from build123d import *
from build123d.topology import SkipClean

# Parameters (mm, degrees)
BASPROSKE_W      = 3
BASPROSKE_H      = 4.25
TOOTHCUT_DEPTH   = 7.717514421
TEETHCUTS_COUNT  = 15
TEETHCUTS_ANGLE  = 336
HUBNEARONE_START = 2.0000508
HUBNEAONESKE_R   = 3.124
HUBNEARONE_DEPTH = 2.0000508
BORSKE_R         = 1.75
BORE_DEPTH       = 5.0000508


with BuildPart() as part:
    # BasProSke → Base-Revolve (revolve)
    with BuildSketch(Plane(origin=(0, 0, 0), x_dir=(1, 0, 0), z_dir=(0, 1, 0)), mode=Mode.PRIVATE) as base_revolve_sk:
        with Locations((1.5, 2.125)):
            Rectangle(BASPROSKE_W, BASPROSKE_H)
    revolve(base_revolve_sk.sketch.rotate(Axis((-10, 0, 0), (1, 0, 0)), 180), axis=Axis((-10, 0, 0), (1, 0, 0)))

    # TooCutSke → ToothCut (cut, through all)
    with BuildSketch(Plane(origin=(0, 0, 0), x_dir=(0, 0, -1), z_dir=(1, 0, 0))):
        with BuildLine():
            ThreePointArc((0.265767165, 3.112674704), (0, 3.124), (-0.265767165, 3.112674704))
            ThreePointArc((-0.265767165, 3.112674704), (-0.418628877, 3.712626775), (-0.800767345, 4.19974009))
            ThreePointArc((-0.800767345, 4.19974009), (0, 4.2754), (0.800767345, 4.19974009))
            ThreePointArc((0.800767345, 4.19974009), (0.418628877, 3.712626775), (0.265767165, 3.112674704))
        make_face()
    toothcut = extrude(amount=TOOTHCUT_DEPTH, mode=Mode.SUBTRACT)

    # TeethCuts: ToothCut ×15 about axis
    teethcuts_axis = Axis((-10, 0, 0), (1, 0, 0))
    for i in range(1, TEETHCUTS_COUNT):
        add(toothcut.rotate(teethcuts_axis, i * TEETHCUTS_ANGLE / (TEETHCUTS_COUNT - 1)), mode=Mode.SUBTRACT)

    # HubNeaOneSke → HubNearOne (add)
    with SkipClean():  # the faces are left unmerged after this step: merging them gives an invalid solid
        with BuildSketch(Plane.ZY.offset(HUBNEARONE_START)):
            Circle(HUBNEAONESKE_R)
        extrude(amount=-HUBNEARONE_DEPTH)

    # BorSke → Bore (cut, symmetric)
    with SkipClean():  # the faces are left unmerged after this step: merging them gives an invalid solid
        with BuildSketch(Plane(origin=(0, 0, 0), x_dir=(0, 0, -1), z_dir=(1, 0, 0))):
            with Locations(Location((0, 0, 0), (0, 0, 180))):
                Circle(BORSKE_R)
        extrude(amount=BORE_DEPTH, both=True, mode=Mode.SUBTRACT)


solid = part.part
Geometry: final body of the model. Coordinates: model frame, mm. A direction names the side the tool comes from. Give positions to 0.01 mm unless a question says otherwise; leave off trailing zeros. Write each loop counter-clockwise with the first axis right and the second up, starting at its lowest first coordinate (ties: lowest second). Pieces come first, ordered by that corner, then holes.
(1) Cut plane B-B, the plane x = -0.2. Return loops of the section in (y, z).
(2) First-contact query: P1, Ø1.5, axis at x = -1, z = -3, coming from the +Y side; P2, Ø0.5, axis at y = 3, z = 2, coming from the -X side; P3, Ø1, axis at x = 0, y = -3.5, coming from the +Z side. Flat tips, straight axial feed; report the tip coordinate or a pass-through.
(3) Access query for faces 1 (the flat face through (0, 2, 3)), 2 (the cylindrical face through (1.48, -3.54, 1.18)), 3 (the cylindrical face through (1.48, 3.22, -1.89)), 4 (the cylindrical face through (1.48, 2.77, -2.47)), 5 (the cylindrical face through (1.479, -3.711, -0.364)). Directions: +Z, -Z, +X, -X, +Y, -Y. A direction counts if a zero-diameter tool reaches every point of the face in a straight line with its end or side. Return the directions, or none.
(4) Mould query, pull axis Z, two halves, no side actions, for faces 6 (the flat face through (0, -2.4, 2.6)), 7 (the cylindrical face through (1.479, -2.198, 2.992)), 8 (the cylindrical face through (1.48, -3.23, 1.84)). Classes: released by +Z, released by -Z, zero draft, split by the parting line, or undercut.
(5) Ray query, line 1 (Y direction, x = 1.35, z = 3.5); line 2 (Z direction, x = 2.6, y = -3.25); line 3 (Y direction, x = -0.15, z = 0). Return the intervals inside material, ascending.
(6) Cut plane A-A, the plane z = 0. Return loops of the section in (x, y), then the cut area to 3 significant figures.
(7) Cut plane C-C, the plane z = 2.25. Return loops of the section in (x, y), then the cut area to 3 significant figures.
Values follow:
1. outline: circle Ø6.25 at (0, 0); hole circle Ø3.5 at (0, 0)
2. P1: stops at y = 2.17
2. P2: stops at x = 0
2. P3: stops at z = 1.87
3. face 1: +Z, -X, +Y
3. face 2: +X, -X, -Y
3. face 3: +X, -X, +Y
3. face 4: -Z, +X, -X
3. face 5: +X, -X
4. face 6: zero draft
4. face 7: released by +Z
4. face 8: undercut
5. line 1: y = -1.5 to -0.72, -0.04 to 0.76, 1.65 to 2.23
5. line 2: z = -1.84 to -1, -0.4 to 0.4, 1 to 1.84
5. line 3: y = -3.12 to -1.75, 1.75 to 3.12
6. outline: (-2, -3.12) - (0, -3.12) - (0, -4.25) - (3, -4.25) - (3, -1.75) - (-2, -1.75) - close; (-2, 1.75) - (3, 1.75) - (3, 3.12) - (-2, 3.12) - close
6. area: 17.1 mm2
7. outline: (-2, -2.17) - (0, -2.17) - (0, -2.57) - (3, -2.57) - (3, 2.17) - (-2, 2.17) - close; (0, 2.41) - (3, 2.41) - (3, 3.44) - (0, 3.44) - close
7. area: 26.0 mm2
